Geometry: final body of the model. Coordinates: model frame, mm. A direction names the side the tool comes from. Round coordinates to 2 decimals unless told otherwise and drop trailing zeros. Loops run counter-clockwise (first coordinate to the right, second up) from the corner with the lowest first, then second, coordinate; pieces in that order, holes last. Notation, with made-up numbers: M 54.25,73 L 99.25,73 A24 cw 99.25,96 Z; hole C -23.75,-4.75 d1. An arc over 180 degrees is marked long. Write each question's results on one line, items separated by ' | '.
```python
from build123d import *

# Parameters (mm, degrees)
F0_R     = 10
F0_R_2   = 8.5
F1_DEPTH = 3
F3_DEPTH = 1.3


with BuildPart() as f1:
    # F0 (on Top) → F1 (new body)
    with BuildSketch(Plane.XY):
        Circle(F0_R)
        Circle(F0_R_2, mode=Mode.SUBTRACT)
    extrude(amount=F1_DEPTH)

    # F2 (on face) → F3 (cut)
    with BuildSketch(Plane(origin=(0, 0, 0), x_dir=(1, 0, 0), z_dir=(0, 0, -1))):
        with BuildLine():
            ThreePointArc((0.95, 9.954773), (0, 10), (-0.95, 9.954773))
            Line((-0.95, 9.954773), (-0.95, 8.446745))
            ThreePointArc((-0.95, 8.446745), (0, 8.5), (0.95, 8.446745))
            Line((0.95, 8.446745), (0.95, 9.954773))
        make_face()
        with BuildLine():
            ThreePointArc((-0.95, -9.954773), (0, -10), (0.95, -9.954773))
            Line((0.95, -9.954773), (0.95, -8.446745))
            ThreePointArc((0.95, -8.446745), (0, -8.5), (-0.95, -8.446745))
            Line((-0.95, -8.446745), (-0.95, -9.954773))
        make_face()
    extrude(amount=-F3_DEPTH, mode=Mode.SUBTRACT)


solid = f1.part
```
1. Section A-A (x = 0). Output: boundary loops of the cut face in (y, z), then the cut area to 3 significant figures.
Answer key:
outline: M -10,1.3 L -8.5,1.3 L -8.5,3 L -10,3 Z; M 8.5,1.3 L 10,1.3 L 10,3 L 8.5,3 Z | area: 5.10 mm²
2. Pin query (flat end, axial travel): P1, Ø1.2, axis at x = 0, y = -9.5, coming from the -Z side; P2, Ø1.5, axis at y = 7, z = 1.5, coming from the -X side; P3, Ø1, axis at y = 9, z = 1, coming from the -X side. Return the tip coordinate at first contact, or that it passes through.
Answer key:
P1: stops at z = 1.3 | P2: stops at x = -7.81 | P3: stops at x = -5.27
3. Access query for faces 4 (the face through (0, 9, 1.3)), 5 (the face through (-9, 0, 0)). Directions: +Z, -Z, +X, -X, +Y, -Y. A direction counts if a zero-diameter tool reaches every point of the face in a straight line with its end or side. Return the directions, or none.
Answer key:
face 4: -Z, +Y, -Y | face 5: -Z, +X, -X, +Y, -Y
4. Section C-C (z = 2). Output: boundary loops of the cut face in (x, y).
Answer key:
outline: C 0,0 d20; hole C 0,0 d17
5. Ray query, probe 1 along Y at (x, z) = (0, 2.1); probe 2 along X at (y, z) = (2.75, 2). Return the intervals inside material, ascending.
Answer key:
probe 1: y = -10 to -8.5, 8.5 to 10 | probe 2: x = -9.61 to -8.04, 8.04 to 9.61
6. Draft query along Y for faces 1 (the face through (4.57, 7.167, 1.479)), 2 (the face through (-2.17, -9.76, 1.48)), 3 (the face through (-4.5, -7.4, 3)). Return one class per face: pulls with the +Y half, pulls with the -Y half, needs draft (parallel to the pull), parting line crosses it, or undercut.
Answer key:
face 1: undercut | face 2: parting line crosses it | face 3: needs draft
7. Section B-B (y = 0). Output: boundary loops of the cut face in (x, z), then the cut area to 3 significant figures.
Answer key:
outline: M -10,0 L -8.5,0 L -8.5,3 L -10,3 Z; M 8.5,0 L 10,0 L 10,3 L 8.5,3 Z | area: 9.00 mm²
